Autodesk Inventor part; units mm, degrees
ref_plane "YZ Plane" through (0, 0, 0) normal (1, 0, 0) x (0, 1, 0)
ref_plane "XZ Plane" through (0, 0, 0) normal (0, 1, 0) x (-1, 0, 0)
ref_plane "XY Plane" through (0, 0, 0) normal (0, 0, 1) x (1, 0, 0)
sketch "Boceto1" plane through (0, 0, 0) normal (0, 1, 0) x (-1, 0, 0)
  line L0 (0, 0) -> (900, 0)
  line L1 (900, 0) -> (900, -1200)
  line L2 (900, -1200) -> (0, -1200)
  line L3 (0, -1200) -> (0, 0)
  dimension "d0" = 900
  dimension "d1" = 1200
extrude "Extrusión1" add sketch "Boceto1" along normal blind 3
sketch "Boceto2" plane through (0, 3, 0) normal (0, 1, 0) x (1, 0, 0)
  line L0 (0, 1200) -> (-900, 1200)
  line L1 (0, 0) -> (-900, 0)
  line L2 (-900, 0) -> (-900, 1200)
  line L3 (-900, 1200) -> (0, 1200)
  line L4 (0, 1200) -> (0, 0)
  line L5 (-897, 1197) -> (-897, 3)
  line L6 (-897, 3) -> (-3, 3)
  line L7 (-3, 3) -> (-3, 1197)
  line L8 (-3, 1197) -> (-897, 1197)
  dimension "d4" = 3
extrude "Extrusión2" add sketch "Boceto2" along normal blind 50
sketch "Boceto3" plane through (0, 0, -1200) normal (0, 0, -1) x (-1, 0, 0)
  circle A0 centre (52, 28) radius 4
  line L0 (0, 53) -> (900, 53)
  line L1 (0, 53) -> (-3, 53)
  line L2 (-3, 53) -> (-3, -10.4752)
  line L3 (-3, -10.4752) -> (0, -10.4752)
  line L4 (0, -10.4752) -> (0, 53)
  point P0 (0, 0)
  dimension "d7" = 8
  dimension "d8" = 25
  dimension "d9" = 3
  dimension "d10" = 55
extrude "Extrusión3" cut sketch "Boceto3" against normal blind 1243.5 contours A0
properties part number "tapa mesa"
Could you check a few things on this model? Use its own coordinates, in mm. A direction names the side the tool comes from. Give positions to 0.01 mm unless a question says otherwise; leave off trailing zeros. Order: outer loops, then holes, each group sorted by start corner. A loop starts at its lowest first (then second) coordinate and runs counter-clockwise, first axis right, second up.
Q1. Suppose I cut it at B-B, the plane x = -180. Write out the boundary of the cut face in (y, z).
Q2. Suppose I cut it at A-A, the plane z = -597.5. Write out the boundary of the cut face in (x, y).
Q3. We'd pull the mould along Z, two halves only. Please class faces 3 (the flat face through (-444, 26, 0)), 4 (the flat face through (-3, 28, -592)), 5 (the flat face through (-444, 0, -592)): +Z half, -Z half, draft (parallel to the pull), parting line (faces both ways), or undercut.
Q4. I'm going to push a flat-ended pin straight in: P1, Ø4, axis at x = -504.5, z = -420, coming from the +Y side. Where does the tip first touch, or does it pass through?
Q5. If I drill on line 1 along Y through (x, z) = (-52, -1.65); line 2 along Z through (x, y) = (-444.5, 21.5); line 3 along X through (y, z) = (42, -365.5), over which ranges is the centre line in solid material (lowest first)?
Q6. For faces 1 (the flat face through (0, 26, -608)), 2 (the flat face through (-897, 28, -608)), which set-ups out of +Z, -Z, +X, -X, +Y, -Y let a thin tool reach every point of the face, with its end or its side?
Solution:
1. outline: (0, -1200) - (53, -1200) - (53, -1197) - (3, -1197) - (3, -3) - (53, -3) - (53, 0) - (0, 0) - close
2. outline: (-900, 0) - (0, 0) - (0, 53) - (-3, 53) - (-3, 3) - (-897, 3) - (-897, 53) - (-900, 53) - close
3. face 3: +Z half
3. face 4: undercut
3. face 5: draft
4. P1: stops at y = 3
5. line 1: y = 0 to 24, 32 to 53
5. line 2: z = -1200 to -1197, -3 to 0
5. line 3: x = -900 to -897, -3 to 0
6. face 1: +Z, -Z, +X, +Y, -Y
6. face 2: +Y
